```python
from build123d import *

# Parameters (mm, degrees)
SKETCH_1_R      = 2
EXTRUDE_1_DEPTH = 1.2
SKETCH_5_W      = 35
SKETCH_5_H      = 50
EXTRUDE_2_DEPTH = 29
FILLET_1_R      = 3


with BuildPart() as part:
    # 草图1 → 拉伸1 (new body)
    with BuildSketch(Plane.XY):
        with BuildLine():
            Line((-11.958260743, 25), (-17.5, 25))
            Line((-17.5, 25), (-17.5, -25))
            Line((-17.5, -25), (-11.958260743, -25))
            ThreePointArc((-11.958260743, -25), (-7.896241541, -26.584119567), (-5.979130372, -30.5))
            ThreePointArc((-5.979130372, -30.5), (0, -36), (5.979130372, -30.5))
            ThreePointArc((5.979130372, -30.5), (7.896241541, -26.584119567), (11.958260743, -25))
            Line((11.958260743, -25), (17.5, -25))
            Line((17.5, -25), (17.5, 25))
            Line((17.5, 25), (11.958260743, 25))
            ThreePointArc((11.958260743, 25), (7.896241541, 26.584119567), (5.979130372, 30.5))
            ThreePointArc((5.979130372, 30.5), (0, 36), (-5.979130372, 30.5))
            ThreePointArc((-5.979130372, 30.5), (-7.896241541, 26.584119567), (-11.958260743, 25))
        make_face()
        with Locations((0, 30)):
            Circle(SKETCH_1_R, mode=Mode.SUBTRACT)
        with Locations(Location((0, -30, 0), (0, 0, 180))):
            Circle(SKETCH_1_R, mode=Mode.SUBTRACT)
    extrude(amount=EXTRUDE_1_DEPTH)

    # 草图5 → 拉伸2 (add)
    with BuildSketch(Plane.XY.offset(1.2)):
        Rectangle(SKETCH_5_W, SKETCH_5_H)
    extrude(amount=EXTRUDE_2_DEPTH)

    # 圆角1
    fillet_1_edges = [part.edges().sort_by_distance(p)[0] for p in [
        (17.5, 25, 15.1),
        (17.5, -25, 15.1),
        (-17.5, -25, 15.1),
        (-17.5, 25, 15.1),
        (-17.5, 0, 30.2),
        (0, -25, 30.2),
        (17.5, 0, 30.2),
        (0, 25, 30.2),
    ]]
    fillet(fillet_1_edges, radius=FILLET_1_R)


solid = part.part
```
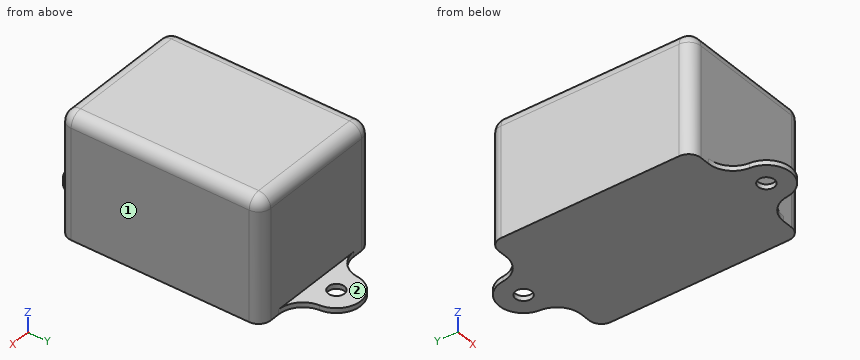
For this review, take the finished solid that the model builds, in its own axes (mm). Face numbers are marked on the shaded views. A direction names the side the tool comes from. Round coordinates to 2 decimals unless told otherwise and drop trailing zeros. Loops run counter-clockwise (first coordinate to the right, second up) from the corner with the lowest first, then second, coordinate; pieces in that order, holes last.
(1) Wall thickness on line 1 along Y through (x, z) = (-5.5, 25.5); line 2 along Z through (x, y) = (-5.5, 29); line 3 along X through (y, z) = (-30, 0.65): over which ranges is each line inside the solid? List them lowest first.
Returned:
line 1: y = -25 to 25
line 2: z = 0 to 1.2
line 3: x = -6.04 to -2, 2 to 6.04
(2) We need section A-A (x = 0). Give the boundary of the cut face in (y, z).
Returned:
outline: (-36, 0) - (-32, 0) - (-32, 1.2) - (-36, 1.2) - close; (-28, 0) - (28, 0) - (28, 1.2) - (25, 1.2) - (25, 27.2) arc R3 ccw to (22, 30.2) - (-22, 30.2) arc R3 ccw to (-25, 27.2) - (-25, 1.2) - (-28, 1.2) - close; (32, 0) - (36, 0) - (36, 1.2) - (32, 1.2) - close
(3) We need section B-B (z = 24). Give the boundary of the cut face in (x, y).
Returned:
outline: (-17.5, -22) arc R3 ccw to (-14.5, -25) - (14.5, -25) arc R3 ccw to (17.5, -22) - (17.5, 22) arc R3 ccw to (14.5, 25) - (-14.5, 25) arc R3 ccw to (-17.5, 22) - close
(4) Tool access review of the marked faces 1 and 2: name each direction out of +Z, -Z, +X, -X, +Y, -Y from which nothing blocks a thin tool from reaching the whole face with its end or side.
Returned:
face 1: +Z, -Z, +X, +Y, -Y
face 2: +Z, +X, -X, +Y
(5) Clearance check with flat-ended pins moving along their axes: P1, Ø3, axis at x = -7.5, z = 26.5, coming from the -Y side; P2, Ø9, axis at x = -1, y = -31.5, coming from the +Z side; P3, Ø13.5, axis at x = -2.5, z = 8, coming from the +Y side. State where each tip first meets the part, or that it passes through.
Returned:
P1: stops at y = -25
P2: stops at z = 1.2
P3: stops at y = 25
(6) We need section D-D (x = -3.5). Give the boundary of the cut face in (y, z).
Returned:
outline: (-34.87, 0) - (34.87, 0) - (34.87, 1.2) - (25, 1.2) - (25, 27.2) arc R3 ccw to (22, 30.2) - (-22, 30.2) arc R3 ccw to (-25, 27.2) - (-25, 1.2) - (-34.87, 1.2) - close
(7) We need section C-C (x = -13.5). Give the boundary of the cut face in (y, z), plus the area to 3 significant figures.
Returned:
outline: (-25, 0) - (25, 0) - (25, 27.2) arc R3 ccw to (22, 30.2) - (-22, 30.2) arc R3 ccw to (-25, 27.2) - close
area: 1,510 mm2
